from build123d import *

# Parameters (mm, degrees)
F0_W     = 25.4
F0_H     = 25.4
F0_R     = 1.5875
F1_DEPTH = 12.7


with BuildPart() as f1:
    # F0 (on Top) → F1 (new body)
    with BuildSketch(Plane.XY):
        Polygon((44.45, -6.35), (57.15, -6.35), (57.15, 6.35), (-57.15, 6.35), (-57.15, -6.35), (-31.75, -6.35), (31.75, -6.35), align=None)
        with Locations((-44.45, -19.05)):
            Rectangle(F0_W, F0_H)
        with Locations((-44.45, -19.05)):
            Circle(F0_R, mode=Mode.SUBTRACT)
        Polygon((69.85, -6.35), (57.15, -6.35), (44.45, -6.35), (44.45, -31.75), (69.85, -31.75), align=None)
        with Locations((57.15, -19.05)):
            Circle(F0_R, mode=Mode.SUBTRACT)
        Polygon((57.15, 6.35), (57.15, -6.35), (69.85, -6.35), (69.85, 31.75), (57.15, 31.75), align=None)
        with Locations((63.5, 26.9875)):
            Circle(F0_R, mode=Mode.SUBTRACT)
    extrude(amount=F1_DEPTH)


solid = f1.part
Here's how the part is built. I have some questions about the finished solid (model axes, mm). A direction names the side the tool comes from. Round coordinates to 2 decimals unless told otherwise and drop trailing zeros. Loops run counter-clockwise (first coordinate to the right, second up) from the corner with the lowest first, then second, coordinate; pieces in that order, holes last.
1. If we section it at A-A on x = -44.45: Write out the boundary of the cut face in (y, z), plus the area to 3 significant figures.
Answer list:
outline: (-31.75, 0) - (-20.64, 0) - (-20.64, 12.7) - (-31.75, 12.7) - close; (-17.46, 0) - (6.35, 0) - (6.35, 12.7) - (-17.46, 12.7) - close
area: 444 mm2
2. If we section it at C-C on z = 2.75: Count the separate pieces of the cut face and the enclosed holes in it, plus the area to 3 significant figures.
Answer list:
separate pieces: 1
enclosed holes: 3
area: 3,200 mm2
3. If I drill on line 1 along Y through (x, z) = (-44.45, 5.5); line 2 along Y through (x, z) = (63.5, 3) (3 decimals); line 3 along X through (y, z) = (-28.5, 4.25), over which ranges is the centre line in solid material (lowest first)?
Answer list:
line 1: y = -31.75 to -20.64, -17.46 to 6.35
line 2: y = -31.75 to 25.4, 28.575 to 31.75
line 3: x = -57.15 to -31.75, 44.45 to 69.85
4. Which directions (+Z, -Z, +X, -X, +Y, -Y) give clear straight access to the entire face, cutting with the end or side of a thin tool? Please do faces 1 (the face through (-31.75, -19, 6)), 2 (the face through (58, -17.71, 6.26)), 3 (the face through (1, 6.35, 6)).
Answer list:
face 1: +Z, -Z, -Y
face 2: +Z, -Z
face 3: +Z, -Z, -X, +Y
5. If we section it at B-B on y = -19.05: Write out the boundary of the cut face in (x, z), plus the area to 3 significant figures.
Answer list:
outline: (-57.15, 0) - (-46.04, 0) - (-46.04, 12.7) - (-57.15, 12.7) - close; (-42.86, 0) - (-31.75, 0) - (-31.75, 12.7) - (-42.86, 12.7) - close; (44.45, 0) - (55.56, 0) - (55.56, 12.7) - (44.45, 12.7) - close; (58.74, 0) - (69.85, 0) - (69.85, 12.7) - (58.74, 12.7) - close
area: 565 mm2
6. We'd pull the mould along X, two halves only. Please class faces 4 (the face through (-46.036, -18.98, 6.261)), 5 (the face through (-57.15, -12, 6)), 6 (the face through (15, -5, 12.7)): +X half, -X half, draft (parallel to the pull), parting line (faces both ways), or undercut.
Answer list:
face 4: undercut
face 5: -X half
face 6: draft
7. For P1, Ø2, axis at y = 12.5, z = 4.5, coming from the -X side; P2, Ø6, axis at x = -28, z = 10.5, coming from the +Y side, each with a flat end and sliding along its axis, tell me the tip position at first contact or that it passes through.
Answer list:
P1: stops at x = 57.15
P2: stops at y = 6.35
8. If we section it at D-D on x = 63.5: Write out the boundary of the cut face in (y, z) (3 decimals).
Answer list:
outline: (-31.75, 0) - (25.4, 0) - (25.4, 12.7) - (-31.75, 12.7) - close; (28.575, 0) - (31.75, 0) - (31.75, 12.7) - (28.575, 12.7) - close
